For this review, take the finished solid that the model builds, in its own axes (mm). A direction names the side the tool comes from. Round coordinates to 2 decimals unless told otherwise and drop trailing zeros. Write each loop counter-clockwise with the first axis right and the second up, starting at its lowest first coordinate (ties: lowest second). Pieces come first, ordered by that corner, then holes. Notation, with made-up numbers: (30, 55) -> (62, 55) arc R16 ccw to (62, 79) -> close; hole circle Ø1 at (12, 12). An arc over 180 degrees is marked (long way). Answer in a Markdown table with one row per item.
from build123d import *

# Parameters (mm, degrees)
SKETCH_3_W          = 40
SKETCH_3_H          = 30
SKETCH_3_R          = 2.5
EXTRUDE_3_DEPTH     = 8
SKETCH_4_W          = 30
SKETCH_4_H          = 25
SKETCH_4_R          = 2.5
EXTRUDE_4_DEPTH     = 9
SKETCH_5_R          = 4
CUT_EXTRUDE_1_DEPTH = 1
SKETCH_6_R          = 4
CUT_EXTRUDE_2_DEPTH = 1


with BuildPart() as part:
    # 스케치3 → 보스-돌출3 (new body)
    with BuildSketch(Plane(origin=(0, 0, 0), x_dir=(1, 0, 0), z_dir=(0, 1, 0))):
        with Locations((20, -15)):
            Rectangle(SKETCH_3_W, SKETCH_3_H)
        with Locations(Location((20, -15, 0), (0, 0, 270))):
            Circle(SKETCH_3_R, mode=Mode.SUBTRACT)
    extrude(amount=EXTRUDE_3_DEPTH)

    # 스케치4 → 보스-돌출4 (add)
    with BuildSketch(Plane(origin=(0, 0, 0), x_dir=(0, 0, -1), z_dir=(1, 0, 0))):
        with Locations((-15, 12.5)):
            Rectangle(SKETCH_4_W, SKETCH_4_H)
        with Locations((-15, 14)):
            Circle(SKETCH_4_R, mode=Mode.SUBTRACT)
    extrude(amount=EXTRUDE_4_DEPTH)

    # 스케치5 → 컷-돌출1 (cut)
    with BuildSketch(Plane(origin=(0, 8, 0), x_dir=(1, 0, 0), z_dir=(0, 1, 0))):
        with Locations(Location((20, -15, 0), (0, 0, 270))):
            Circle(SKETCH_5_R)
    extrude(amount=-CUT_EXTRUDE_1_DEPTH, mode=Mode.SUBTRACT)

    # 스케치6 → 컷-돌출2 (cut)
    with BuildSketch(Plane(origin=(9, 0, 0), x_dir=(0, 0, -1), z_dir=(1, 0, 0))):
        with Locations((-15, 14)):
            Circle(SKETCH_6_R)
    extrude(amount=-CUT_EXTRUDE_2_DEPTH, mode=Mode.SUBTRACT)


solid = part.part
1) Consider section C-C on y = 14. State the section outline as (x, z) points.
Solved:
| item | result |
|---|---|
| outline | (0, 0) -> (9, 0) -> (9, 11) -> (8, 11) -> (8, 12.5) -> (0, 12.5) -> close; (0, 17.5) -> (8, 17.5) -> (8, 19) -> (9, 19) -> (9, 30) -> (0, 30) -> close |
2) Consider section D-D on x = 5. State the section outline as (y, z) points, then the cut area to 3 significant figures.
Solved:
| item | result |
|---|---|
| outline | (0, 0) -> (25, 0) -> (25, 30) -> (0, 30) -> close; hole circle Ø5 at (14, 15) |
| area | 730 mm² |
3) Clearance check with flat-ended pins moving along their axes: pin 1 Ø4 at (y, z) = (14, 12) entering from +X; pin 2 Ø10.5 at (x, z) = (20, 15) entering from +Y; pin 3 Ø1.5 at (x, z) = (22.5, 13.5) entering from +Y; pin 4 Ø4 at (y, z) = (14, 15) entering from +X. State where each tip first meets the part, or that it passes through.
Solved:
| item | result |
|---|---|
| pin 1 | x = 9 |
| pin 2 | y = 8 |
| pin 3 | y = 7 |
| pin 4 | through |
4) Consider section B-B on z = 15. State the section outline as (x, y) points, then the cut area to 3 significant figures.
Solved:
| item | result |
|---|---|
| outline | (0, 0) -> (17.5, 0) -> (17.5, 7) -> (16, 7) -> (16, 8) -> (9, 8) -> (9, 10) -> (8, 10) -> (8, 11.5) -> (0, 11.5) -> close; (0, 16.5) -> (8, 16.5) -> (8, 18) -> (9, 18) -> (9, 25) -> (0, 25) -> close; (22.5, 0) -> (40, 0) -> (40, 8) -> (24, 8) -> (24, 7) -> (22.5, 7) -> close |
| area | 382 mm² |
5) Consider section A-A on x = 20. State the section outline as (y, z) points, then the cut area to 3 significant figures.
Solved:
| item | result |
|---|---|
| outline | (0, 0) -> (8, 0) -> (8, 11) -> (7, 11) -> (7, 12.5) -> (0, 12.5) -> close; (0, 17.5) -> (7, 17.5) -> (7, 19) -> (8, 19) -> (8, 30) -> (0, 30) -> close |
| area | 197 mm² |
6) For line 1 (Z direction, x = 20, y = 3.25); line 2 (Y direction, x = 8.7, z = 15); line 3 (Y direction, x = 5.25, z = 15), list the stretches that pass through material, from the lowest coordinate up. Write a range as [from, to].
Solved:
| item | result |
|---|---|
| line 1 | [0, 12.5], [17.5, 30] |
| line 2 | [0, 10], [18, 25] |
| line 3 | [0, 11.5], [16.5, 25] |
7) For faces 4 (the flat face through (18, 7, 13)), 5 (the flat face through (24.3, 8, 14.8)), 6 (the flat face through (8, 12, 17)), list the 3-axis set-ups (+Z, -Z, +X, -X, +Y, -Y) from which the entire face can be reached by the end or side of a thin tool; tool diameter is ignored.
Solved:
| item | result |
|---|---|
| face 4 | +Y |
| face 5 | +Z, -Z, +X, +Y |
| face 6 | +X |
8) Mouldability with a two-part tool opening along Z and no side actions: class faces 1 (the flat face through (15, 7, 30)), 2 (the cylindrical face through (8.507, 14.176, 18.996)), 3 (the flat face through (40, 4, 15)) as pulls with the +Z half, pulls with the -Z half, needs draft (parallel to the pull), parting line crosses it, or undercut.
Solved:
| item | result |
|---|---|
| face 1 | pulls with the +Z half |
| face 2 | undercut |
| face 3 | needs draft |
